```python
from build123d import *

# Parameters (mm, degrees)
F0_R     = 57.5
F1_DEPTH = 36
F2_R     = 53.5
F3_DEPTH = 7
F4_R     = 45
F5_DEPTH = 29.001


with BuildPart() as f1:
    # F0 (on Front) → F1 (new body)
    with BuildSketch(Plane.XZ):
        Circle(F0_R)
    extrude(amount=F1_DEPTH)

    # F2 (on face) → F3 (cut)
    with BuildSketch(Plane.XZ.offset(36)):
        Circle(F2_R)
    extrude(amount=-F3_DEPTH, mode=Mode.SUBTRACT)

    # F4 (on face) → F5 (cut, through all)
    with BuildSketch(Plane.XZ.offset(29)):
        Circle(F4_R)
    extrude(amount=-F5_DEPTH, mode=Mode.SUBTRACT)


solid = f1.part
```
Input: part model. Units: mm. Frame: model coordinates. Coordinates: 2 decimals unless noted, no trailing zeros. Write each loop counter-clockwise with the first axis right and the second up, starting at its lowest first coordinate (ties: lowest second). Pieces come first, ordered by that corner, then holes. Notation, with made-up numbers: (79, 2) -> (97, 2) arc R28 ccw to (97, 35) -> close; hole circle Ø5 at (85.25, 40). An arc over 180 degrees is marked (long way). Answer as a JSON object with one key per item and string values.
1. Section A-A on z = 0. Return the cut outline in (x, y), then the cut area to 3 significant figures.
Result set:
{"outline": "(-57.5, -36) -> (-53.5, -36) -> (-53.5, -29) -> (-45, -29) -> (-45, 0) -> (-57.5, 0) -> close; (45, -29) -> (53.5, -29) -> (53.5, -36) -> (57.5, -36) -> (57.5, 0) -> (45, 0) -> close", "area": "781 mm2"}
2. Mould query, pull axis Z, two halves, no side actions, for faces 1 (the face through (-12, -29, 44)), 2 (the face through (-34, 0, -30)), 3 (the face through (-12.465, -17.748, -56.133)), 4 (the face through (-11.598, -32.549, -52.228)). Classes: released by +Z, released by -Z, zero draft, split by the parting line, or undercut.
Result set:
{"face 1": "undercut", "face 2": "zero draft", "face 3": "split by the parting line", "face 4": "undercut"}
3. Material intervals for line 1 (Z direction, x = 0, y = -34); line 2 (Z direction, x = 0, y = -6.25); line 3 (Y direction, x = -37, z = 27), sorted ascending. Write a range as from..to.
Result set:
{"line 1": "z = -57.5..-53.5, 53.5..57.5", "line 2": "z = -57.5..-45, 45..57.5", "line 3": "y = -29..0"}
4. First-contact query: P1, Ø12, axis at y = -21.5, z = 22, coming from the +X side; P2, Ø5, axis at x = 33.5, z = 33.5, coming from the -Y side; P3, Ø8, axis at y = -25, z = -9.5, coming from the +X side; P4, Ø10, axis at y = -12.5, z = 4.5, coming from the +X side. Flat tips, straight axial feed; report the tip coordinate or a pass-through.
Result set:
{"P1": "stops at x = 55.23", "P2": "stops at y = -29", "P3": "stops at x = 57.24", "P4": "stops at x = 57.5"}
5. Section B-B on x = 0. Return the cut outline in (y, z), then the cut area to 3 significant figures.
Result set:
{"outline": "(-36, -57.5) -> (0, -57.5) -> (0, -45) -> (-29, -45) -> (-29, -53.5) -> (-36, -53.5) -> close; (-36, 53.5) -> (-29, 53.5) -> (-29, 45) -> (0, 45) -> (0, 57.5) -> (-36, 57.5) -> close", "area": "781 mm2"}
6. Section C-C on y = -21.5. Return the cut outline in (x, z), then the cut area to 3 significant figures.
Result set:
{"outline": "circle Ø115 at (0, 0); hole circle Ø90 at (0, 0)", "area": "4,030 mm2"}
